Geometry check sheet. Reference: the model listing, model coordinates, mm. A direction names the side the tool comes from. Coordinates: 2 decimals unless noted, no trailing zeros. Write each loop counter-clockwise with the first axis right and the second up, starting at its lowest first coordinate (ties: lowest second). Pieces come first, ordered by that corner, then holes. Notation, with made-up numbers: (-39.75, 9) -> (-24.75, 9) arc R26 cw to (-24.75, 40) -> close; hole circle Ø11 at (-14.75, 28.25). An arc over 180 degrees is marked (long way). Answer in a Markdown table with one row per item. Add a question column.
Q1. Section check B-B, the plane y = 3.75. Count the separate pieces of the cut face and the enclosed holes in it, and give its area (3 significant figures).
Q2. Release check for a two-part mould opening along X. For faces 1 (the face through (-4.3, 4.1, -6)), 2 (the face through (-6, 4, -6.269)), 3 (the face through (0.017, 4, -2)), 4 (the face through (-1.682, 4.056, -6.984)) record: pulls with the +X half, pulls with the -X half, needs draft (parallel to the pull), parting line crosses it, or undercut.
Q3. Section check A-A, the plane z = -1.75. Record the boundary of the cut face in (x, y), and give its area (3 significant figures).
Q4. Thickness scan on line 1 (X direction, y = 6.25, z = -0.75); line 2 (Z direction, x = 1.7, y = 4); line 3 (X direction, y = 6.5, z = -6.5). Record the ranges inside material, lowest first.
Q5. Gauge pin test, flat ends, axial feed: P1, Ø3, axis at x = -2, z = -1, coming from the -Y side; P2, Ø0.6, axis at x = -6, y = 3, coming from the +Z side; P3, Ø1.8, axis at y = 3.5, z = -4.5, coming from the +X side. Record the tip position at first contact, or that the pin passes through.
Q6. Section check C-C, the plane x = 0.25. Record the boundary of the cut face in (y, z), and give its area (3 significant figures).
Q7. Tool access check on faces 5 (the face through (-3.983, 4, -2)), 6 (the face through (-6.983, 4, -7)), 7 (the face through (3.517, 4, -2)), 8 (the face through (2, 3, -6)). Record the directions out of +Z, -Z, +X, -X, +Y, -Y that give a thin tool (end or side, any length) a straight path to the whole face; none if there is none.
Q8. Section check D-D, the plane z = -4.75. Record the boundary of the cut face in (x, y).
Autodesk Inventor part; units mm, degrees
ref_plane "YZ Plane" through (0, 0, 0) normal (1, 0, 0) x (0, 1, 0)
ref_plane "XZ Plane" through (0, 0, 0) normal (0, 1, 0) x (-1, 0, 0)
ref_plane "XY Plane" through (0, 0, 0) normal (0, 0, 1) x (1, 0, 0)
sketch "Sketch1" plane through (0, 0, 0) normal (0, 1, 0) x (-1, 0, 0)
  line L0 (1.9826, -0.2694) -> (1.9826, -7.2694)
  line L1 (1.9826, -7.2694) -> (-0.0174, -7.2694)
  line L2 (-0.0174, -7.2694) -> (-0.0174, -0.2694)
  line L3 (-0.0174, -0.2694) -> (-3.5174, -0.2694)
  line L4 (-3.5174, -0.2694) -> (-3.5174, -8.2694)
  line L5 (-3.5174, -8.2694) -> (3.9826, -8.2694)
  line L6 (3.9826, -8.2694) -> (3.9826, -0.2694)
  line L7 (3.9826, -0.2694) -> (1.9826, -0.2694)
  line L8 (-3.5174, -8.2694) -> (-7.5174, -8.2694)
  line L9 (-7.5174, -8.2694) -> (-7.5174, -4.2694)
  line L10 (-7.5174, -4.2694) -> (-3.5174, -4.2694)
  line L11 (-3.5174, -4.2694) -> (-3.5174, -8.2694)
  line L12 (3.9826, -8.2694) -> (6.9826, -8.2694)
  line L13 (6.9826, -8.2694) -> (6.9826, -6.2694)
  line L14 (6.9826, -6.2694) -> (3.9826, -6.2694)
  line L15 (3.9826, -6.2694) -> (3.9826, -8.2694)
  line L16 (-3.5174, -8.2694) -> (-6.5174, -8.2694)
  line L17 (-6.5174, -8.2694) -> (-6.5174, -6.2694)
  line L18 (-6.5174, -6.2694) -> (-3.5174, -6.2694)
  line L19 (-3.5174, -6.2694) -> (-3.5174, -8.2694)
  point P0 (0, 0)
  dimension "d0" = 2
  dimension "d1" = 3.5
  dimension "d2" = 2
  dimension "d5" = 1
  dimension "d6" = 7
  dimension "d7" = 4
  dimension "d8" = 4
  dimension "d18" = 3
  dimension "d19" = 3
  dimension "d24" = 2
extrude "Extrusion1" add sketch "Sketch1" along normal blind 8 contours L7 L6 L5 L4 L3 L2 L1 L0 | L14 L13 L12 L6 | L8 L17 L18 L4
sketch "Sketch2" plane through (7.5174, 0, -8.2694) normal (0, 0, -1) x (-1, 0, 0)
  circle A0 centre (4, 4) radius 2.05
  line L0 (0, 0) -> (0, 8)
  line L1 (1, 8) -> (14.5, 8)
  line L2 (7.5, 0) -> (7.5, 8)
  point P0 (7.5174, 0)
  point P1 (12, 8)
  dimension "d11" = 4.1
  dimension "d12" = 4
  dimension "d13" = 4
  dimension "d17" = 3.5
extrude "Extrusion2" [suppressed]
fillet "Fillet1" radius 1 4 edges at (-1.9826, 4, -7.2694) (0.0174, 4, -7.2694) (3.5174, 4, -6.2694) (-3.9826, 4, -6.2694)
sketch "Sketch3" plane through (3.5174, 0, -0.2694) normal (1, 0, 0) x (0, 0, -1)
  circle A0 centre (4, 4) radius 2
  circle A1 centre (4, 4) radius 1.5
  line L0 (8, 0) -> (8, 8)
  line L1 (0, 0) -> (5, 0)
  point P0 (-0.2694, 0)
  dimension "d20" = 4
  dimension "d21" = 3
  dimension "d22" = 4
  dimension "d23" = 4
extrude "Extrusion3" cut sketch "Sketch3" against normal blind 10 contours A1
extrude "Extrusion4" cut sketch "Sketch3" against normal blind 3.5
extrude "Extrusion5" cut sketch "Sketch3" along normal blind 3.5 contours A0 | A1
properties part number "ethernet card support"
Calculated:
| question | item | result |
|---|---|---|
| 1 | separate pieces | 3 |
| 1 | enclosed holes | 0 |
| 1 | area | 38.8 mm² |
| 2 | face 1 | pulls with the -X half |
| 2 | face 2 | needs draft |
| 2 | face 3 | undercut |
| 2 | face 4 | undercut |
| 3 | outline | (-3.98, 0) -> (-1.98, 0) -> (-1.98, 8) -> (-3.98, 8) -> close; (0.02, 0) -> (3.52, 0) -> (3.52, 8) -> (0.02, 8) -> close |
| 3 | area | 44.0 mm² |
| 4 | line 1 | x = -3.98 to -1.98, 0.02 to 3.52 |
| 4 | line 2 | z = -8.27 to -6.27, -2.27 to -0.27 |
| 4 | line 3 | x = -6.98 to -1.96, -0.01 to 6.52 |
| 5 | P1 | stops at y = 0 |
| 5 | P2 | stops at z = -6.27 |
| 5 | P3 | passes through |
| 6 | outline | (0, -8.27) -> (8, -8.27) -> (8, -0.27) -> (0, -0.27) -> close; hole circle Ø4 at (4, -4.27) |
| 6 | area | 51.4 mm² |
| 7 | face 5 | +Z, -X, +Y, -Y |
| 7 | face 6 | +Z, -Z, -X, +Y, -Y |
| 7 | face 7 | +Z, +X, +Y, -Y |
| 7 | face 8 | +X |
| 8 | outline | (-3.98, 0) -> (-1.98, 0) -> (-1.98, 2.58) -> (-3.98, 2.58) -> close; (-3.98, 5.42) -> (-1.98, 5.42) -> (-1.98, 8) -> (-3.98, 8) -> close; (0.02, 0) -> (3.52, 0) -> (3.52, 2.06) -> (0.02, 2.06) -> close; (0.02, 5.94) -> (3.52, 5.94) -> (3.52, 8) -> (0.02, 8) -> close |
